Can you work these out from the model? Positions are in its coordinate system, mm. A direction names the side the tool comes from. Give positions to 0.01 mm unless a question says otherwise; leave off trailing zeros. Write each loop counter-clockwise with the first axis right and the second up, starting at its lowest first coordinate (ties: lowest second). Pieces come first, ordered by that corner, then holes.
```python
from build123d import *

# Parameters (mm, degrees)
SKETCH1_W           = 54.070507504
SKETCH1_H           = 26
SKETCH1_R           = 1.875
SKETCH1_W_2         = 16.75
SKETCH1_H_2         = 22
BOSS_EXTRUDE1_DEPTH = 2


with BuildPart() as part:
    # Sketch1 → Boss-Extrude1 (new body)
    with BuildSketch(Plane.XY):
        with Locations((0, 13)):
            Rectangle(SKETCH1_W, SKETCH1_H)
        with Locations(Location((17.205126876, 13, 0), (0, 0, 180))):
            Circle(SKETCH1_R, mode=Mode.SUBTRACT)
        with Locations((-17.205126876, 13)):
            Circle(SKETCH1_R, mode=Mode.SUBTRACT)
        with Locations((0, 13)):
            Rectangle(SKETCH1_W_2, SKETCH1_H_2, mode=Mode.SUBTRACT)
    extrude(amount=BOSS_EXTRUDE1_DEPTH)


solid = part.part
```
1) Suppose I cut it at B-B on y = 13. Write out the boundary of the cut face in (x, z) (3 decimals).
Values follow:
outline: (-27.035, 0) - (-19.08, 0) - (-19.08, 2) - (-27.035, 2) - close; (-15.33, 0) - (-8.375, 0) - (-8.375, 2) - (-15.33, 2) - close; (8.375, 0) - (15.33, 0) - (15.33, 2) - (8.375, 2) - close; (19.08, 0) - (27.035, 0) - (27.035, 2) - (19.08, 2) - close
2) Suppose I cut it at A-A on x = -4. Write out the boundary of the cut face in (y, z), plus the area to 3 significant figures.
Values follow:
outline: (0, 0) - (2, 0) - (2, 2) - (0, 2) - close; (24, 0) - (26, 0) - (26, 2) - (24, 2) - close
area: 8.00 mm2
3) Suppose I cut it at C-C on z = 1.1. Write out the boundary of the cut face in (x, y) (3 decimals), plus the area to 3 significant figures.
Values follow:
outline: (-27.035, 0) - (27.035, 0) - (27.035, 26) - (-27.035, 26) - close; hole circle Ø3.75 at (-17.205, 13); hole (-8.375, 2) - (8.375, 2) - (8.375, 24) - (-8.375, 24) - close; hole circle Ø3.75 at (17.205, 13)
area: 1,020 mm2
4) If we mould it in two halves opening along Y, with no side actions, what happens to faces 3 (the face through (8.375, 13, 1)), 4 (the face through (0, 0, 1)), 5 (the face through (0, 25, 0)), 6 (the face through (15.473, 13.718, 0.986))? For each: +Y half, -Y half, draft (parallel to the pull), parting line (faces both ways), or undercut.
Values follow:
face 3: undercut
face 4: -Y half
face 5: draft
face 6: undercut
5) Suppose I cut it at D-D on y = 6. Write out the boundary of the cut face in (x, z) (3 decimals), plus the area to 3 significant figures.
Values follow:
outline: (-27.035, 0) - (-8.375, 0) - (-8.375, 2) - (-27.035, 2) - close; (8.375, 0) - (27.035, 0) - (27.035, 2) - (8.375, 2) - close
area: 74.6 mm2
6) Please list where these lines run through material, in increasing order: L1, parallel to Y at x = 8, z = 1.4; L2, parallel to X at y = 23.25, z = 1.45 (3 decimals); L3, parallel to Y at x = -16.5, z = 0.75.
Values follow:
L1: y = 0 to 2, 24 to 26
L2: x = -27.035 to -8.375, 8.375 to 27.035
L3: y = 0 to 11.26, 14.74 to 26
7) For faces 1 (the face through (0, 2, 1)), 2 (the face through (0, 26, 1)), which set-ups out of +Z, -Z, +X, -X, +Y, -Y let a thin tool reach every point of the face, with its end or its side?
Values follow:
face 1: +Z, -Z
face 2: +Z, -Z, +X, -X, +Y
